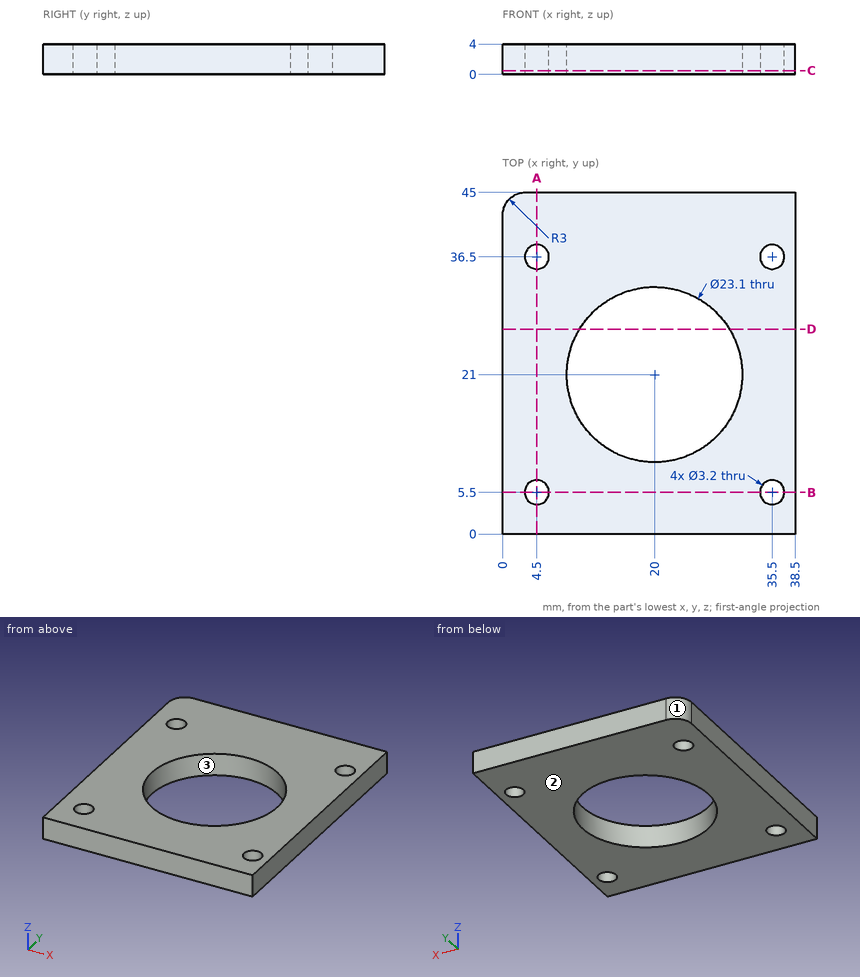
Print and shaded views of the part. All mm, measured from the part's lowest x, y and z. Round coordinates to 2 decimals unless told otherwise and drop trailing zeros. Write each loop counter-clockwise with the first axis right and the second up, starting at its lowest first coordinate (ties: lowest second). Pieces come first, ordered by that corner, then holes.
(1) Slice it at B-B, the plane y = 5.5. Write the cut outline in (x, z).
(2) Probe line 1 along Y through (x, z) = (4.5, 2.05); line 2 along X through (y, z) = (5.5, 1); line 3 along Y through (x, z) = (36.5, 1.75). List the from-to ranges inside material, lowest first.
(3) Mould opens along X. For the marked faces 1, 2 and 3 say: pulls with the +X half, pulls with the -X half, needs draft (parallel to the pull), parting line crosses it, or undercut.
(4) Slice it at A-A, the plane x = 4.5. Write the cut outline in (y, z).
(5) Slice it at D-D, the plane y = 27. Write the cut outline in (x, z).
(6) Slice it at C-C, the plane z = 0.5. Write the cut outline in (x, y), and give its area (3 significant figures).
From the geometry:
1. outline: (0, 0) - (2.9, 0) - (2.9, 4) - (0, 4) - close; (6.1, 0) - (33.9, 0) - (33.9, 4) - (6.1, 4) - close; (37.1, 0) - (38.5, 0) - (38.5, 4) - (37.1, 4) - close
2. line 1: y = 0 to 3.9, 7.1 to 34.9, 38.1 to 45
2. line 2: x = 0 to 2.9, 6.1 to 33.9, 37.1 to 38.5
2. line 3: y = 0 to 4.25, 6.75 to 35.25, 37.75 to 45
3. face 1: pulls with the -X half
3. face 2: needs draft
3. face 3: undercut
4. outline: (0, 0) - (3.9, 0) - (3.9, 4) - (0, 4) - close; (7.1, 0) - (34.9, 0) - (34.9, 4) - (7.1, 4) - close; (38.1, 0) - (45, 0) - (45, 4) - (38.1, 4) - close
5. outline: (0, 0) - (10.13, 0) - (10.13, 4) - (0, 4) - close; (29.87, 0) - (38.5, 0) - (38.5, 4) - (29.87, 4) - close
6. outline: (0, 0) - (38.5, 0) - (38.5, 45) - (3, 45) arc R3 ccw to (0, 42) - close; hole circle Ø3.2 at (4.5, 5.5); hole circle Ø3.2 at (4.5, 36.5); hole circle Ø23.1 at (20, 21); hole circle Ø3.2 at (35.5, 5.5); hole circle Ø3.2 at (35.5, 36.5)
6. area: 1,280 mm2
